Autodesk Inventor part; units mm, degrees
ref_plane "YZ Plane" through (0, 0, 0) normal (1, 0, 0) x (0, 1, 0)
ref_plane "XZ Plane" through (0, 0, 0) normal (0, 1, 0) x (-1, 0, 0)
ref_plane "XY Plane" through (0, 0, 0) normal (0, 0, 1) x (1, 0, 0)
sketch "Sketch1" plane through (0, 0, 0) normal (0, 1, 0) x (-1, 0, 0)
  line L0 (0, 0) -> (-45.2, 0)
  line L1 (-45.2, 0) -> (-45.2, -60.6)
  line L2 (-45.2, -60.6) -> (0, -60.6)
  line L3 (0, -60.6) -> (0, 0)
  dimension "d0" = 45.2
  dimension "d1" = 60.6
extrude "Extrusion1" add sketch "Sketch1" along normal blind 10.58
fillet "Fillet1" radius 10.58 4 edges at (45.2, 5.29, 0) (45.2, 5.29, -60.6) (0, 5.29, -60.6) (0, 5.29, 0)
fillet "Fillet2" radius 10.58 8 edges at (42.1012, 10.58, -57.5012) (22.6, 10.58, -60.6) (3.0988, 10.58, -57.5012) (0, 10.58, -30.3) (3.0988, 10.58, -3.0988) (22.6, 10.58, 0) (42.1012, 10.58, -3.0988) (45.2, 10.58, -30.3)
sketch "Sketch3" plane through (0, 0, 0) normal (0, -1, 0) x (1, 0, 0)
  line L0 (0, 0) -> (-13, 0)
  line L1 (-13, 0) -> (-13, 13)
  line L2 (-13, 13) -> (0, 13)
  line L3 (0, 13) -> (0, 0)
  line L4 (34.62, -50.02) -> (34.62, -10.58)
  line L5 (34.62, -50.02) -> (45.2, -50.02)
  line L6 (45.2, -50.02) -> (45.2, -60.6)
  line L7 (45.2, -60.6) -> (34.62, -60.6)
  line L8 (34.62, -60.6) -> (34.62, -50.02)
  line L9 (45.2, -60.6) -> (58.2, -60.6)
  line L10 (58.2, -60.6) -> (58.2, -73.6)
  line L11 (58.2, -73.6) -> (45.2, -73.6)
  line L12 (45.2, -73.6) -> (45.2, -60.6)
  line L13 (-13, 13) -> (58.2, 13)
  line L14 (58.2, 13) -> (58.2, -73.6)
  line L15 (58.2, -73.6) -> (-13, -73.6)
  line L16 (-13, -73.6) -> (-13, 13)
  dimension "d14" = 13
  dimension "d15" = 13
  dimension "d16" = 13
  dimension "d17" = 13
extrude "Extrusion3" add sketch "Sketch3" along normal blind 3 contours L7 L8 L5 L6 | L3 L13 L14 L9 L12 L15 L16 L0 | L0 L1 L2 L3 | L12 L9 L10 L11
fillet "Fillet4" radius 10.58 4 edges at (-13, -1.5, 13) (-13, -1.5, -73.6) (58.2, -1.5, -73.6) (58.2, -1.5, 13)
properties part number "Airpods Pro Base"
The model under review builds one solid part; all positions refer to its coordinate system, in mm. Round coordinates to 2 decimals unless told otherwise and drop trailing zeros. Write each loop counter-clockwise with the first axis right and the second up, starting at its lowest first coordinate (ties: lowest second). Pieces come first, ordered by that corner, then holes. Notation, with made-up numbers: (58.25, 36) - (91.25, 36) arc R12 ccw to (91.25, 42) - close; hole circle Ø11 at (-7, -11.75). An arc over 180 degrees is marked (long way). One line per item, written item: value. Start each with the question number.
1. Consider section D-D on z = 4. Write out the cut boundary in (x, y), and give its area (3 significant figures).
2. To check wall thickness, follow L1, parallel to Y at x = 52, z = -33; L2, parallel to X at y = -2, z = -67.5; L3, parallel to X at y = 7.25, z = -39. State the ranges of each line that lie inside material, in increasing order. Write a range as from..to.
3. Consider section C-C on x = -6. Write out the cut boundary in (y, z), and give its area (3 significant figures).
4. The part is to be moulded in two halves that separate along X. For faces 1 (the face through (55, -1.5, -70.6)), 2 (the face through (-2, 0, -30)), 3 (the face through (3.02, 7.4, -30.58)), say which applies: released by +X, released by -X, zero draft, split by the parting line, or undercut.
5. Clearance check with flat-ended pins moving along their axes: P1, Ø1.5, axis at y = 6, z = -42.5, coming from the +X side; P2, Ø1.5, axis at y = 8.5, z = -21, coming from the -X side; P3, Ø2, axis at y = 4.5, z = -10, coming from the +X side. State where each tip first meets the part, or that it passes through.
Checks:
1. outline: (-12.88, -3) - (58.08, -3) - (58.08, 0) - (-12.88, 0) - close
1. area: 213 mm^2
2. L1: y = -3..0
2. L2: x = -12..57.2
2. L3: x = 2.87..42.33
3. outline: (-3, -72.98) - (0, -72.98) - (0, 12.38) - (-3, 12.38) - close
3. area: 256 mm^2
4. face 1: released by +X
4. face 2: zero draft
4. face 3: released by -X
5. P1: stops at x = 43.81
5. P2: stops at x = 3.38
5. P3: stops at x = 44.59
